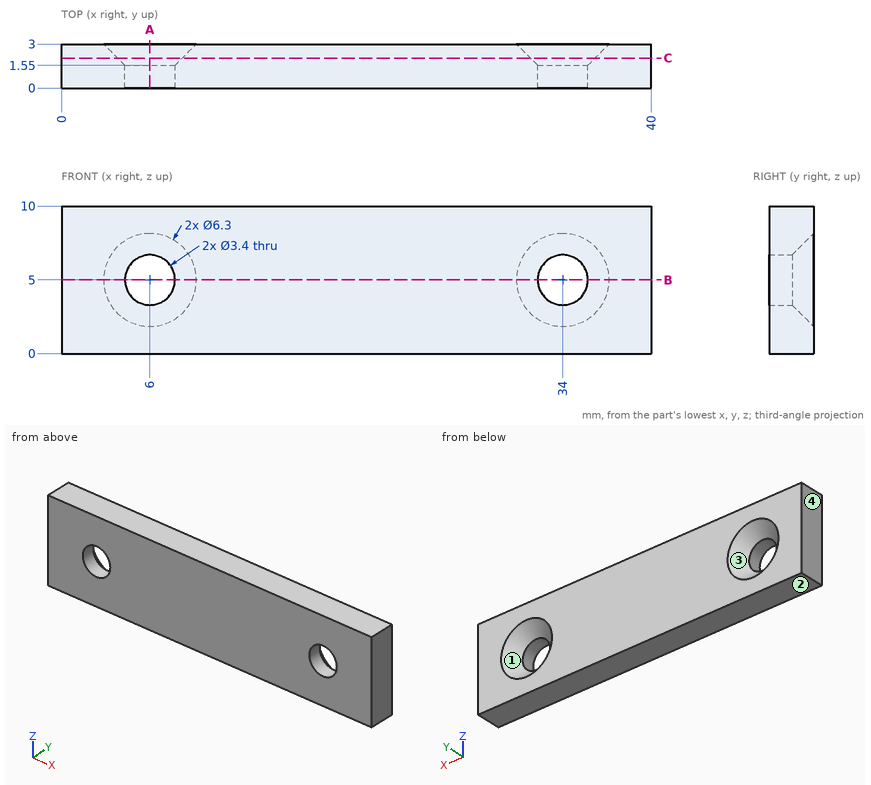
Geometry check sheet. Reference: drawing and pictorial views, mm from the part's lowest x, y, z. Give positions to 0.01 mm unless a question says otherwise; leave off trailing zeros. Order: outer loops, then holes, each group sorted by start corner. A loop starts at its lowest first (then second) coordinate and runs counter-clockwise, first axis right, second up. Notation, with made-up numbers: M 8.25,18 L 50.25,18 A26 ccw 50.25,41 Z; hole C 63,-5 d11. An arc over 180 degrees is marked long. Answer as a JSON object with one key per item and string values. Group by question number.
1) Mould release check, pull along Z, two halves, no side actions. Record for the marked faces 1, 2, 3 and 4: released by +Z, released by -Z, zero draft, split by the parting line, or undercut.
2) Depth check by flat-ended pin: pin 1 Ø1.5 at (x, z) = (4, 5) entering from -Y. Enter the tip coordinate at first touch or a pass-through.
3) Cross-section at B-B (z = 5). Enter the section's corners in (x, y), then the cut area to 3 significant figures.
4) Scan lines: line 1 along X through (y, z) = (0.45, 5); line 2 along Z through (x, y) = (34, 0.95); line 3 along X through (y, z) = (1.8, 5.5). Record each from-to range of solid material in increasing order. Write a range as [from, to].
5) Cross-section at A-A (x = 6). Enter the section's corners in (y, z), then the cut area to 3 significant figures.
6) Cross-section at C-C (y = 2.05). Enter the section's corners in (x, z), then the cut area to 3 significant figures.
Result sheet:
{
 "1": {"face 1": "undercut", "face 2": "released by -Z", "face 3": "undercut", "face 4": "zero draft"},
 "2": {"pin 1": "stops at y = 0"},
 "3": {"outline": "M 0,0 L 4.3,0 L 4.3,1.55 L 2.85,3 L 0,3 Z; M 7.7,0 L 32.3,0 L 32.3,1.55 L 30.85,3 L 9.15,3 L 7.7,1.55 Z; M 35.7,0 L 40,0 L 40,3 L 37.15,3 L 35.7,1.55 Z", "area": "95.4 mm2"},
 "4": {"line 1": "x = [0, 4.3], [7.7, 32.3], [35.7, 40]", "line 2": "z = [0, 3.3], [6.7, 10]", "line 3": "x = [0, 4.12], [7.88, 32.12], [35.88, 40]"},
 "5": {"outline": "M 0,0 L 3,0 L 3,1.85 L 1.55,3.3 L 0,3.3 Z; M 0,6.7 L 1.55,6.7 L 3,8.15 L 3,10 L 0,10 Z", "area": "17.7 mm2"},
 "6": {"outline": "M 0,0 L 40,0 L 40,10 L 0,10 Z; hole C 6,5 d4.4; hole C 34,5 d4.4", "area": "370 mm2"}
}
